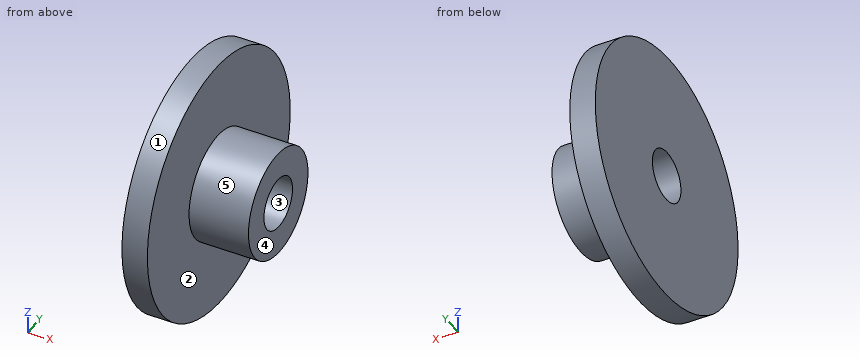
```python
from build123d import *

# Parameters (mm, degrees)
SKETCH1_R           = 30
BOSS_EXTRUDE1_DEPTH = 3
SKETCH2_R           = 12.5
BOSS_EXTRUDE2_DEPTH = 14
SKETCH3_R           = 6
CUT_EXTRUDE1_DEPTH  = 47.904157598


with BuildPart() as part:
    # Sketch1 → Boss-Extrude1 (new, symmetric)
    with BuildSketch(Plane(origin=(0, 0, 0), x_dir=(0, 0, -1), z_dir=(1, 0, 0))):
        Circle(SKETCH1_R)
    extrude(amount=BOSS_EXTRUDE1_DEPTH, both=True)

    # Sketch2 → Boss-Extrude2 (add)
    with BuildSketch(Plane(origin=(3, 0, 0), x_dir=(0, 0, -1), z_dir=(1, 0, 0))):
        Circle(SKETCH2_R)
    extrude(amount=BOSS_EXTRUDE2_DEPTH)

    # Sketch3 → Cut-Extrude1 (cut, through all)
    with BuildSketch(Plane(origin=(17, 0, 0), x_dir=(0, 0, -1), z_dir=(1, 0, 0))):
        Circle(SKETCH3_R)
    extrude(amount=-CUT_EXTRUDE1_DEPTH, mode=Mode.SUBTRACT)


solid = part.part
```
The listing builds one solid part. Answer for the finished solid, in the listing's coordinates (mm). Face numbers are marked on the shaded views. A direction names the side the tool comes from. Round coordinates to 2 decimals unless told otherwise and drop trailing zeros. Order: outer loops, then holes, each group sorted by start corner. A loop starts at its lowest first (then second) coordinate and runs counter-clockwise, first axis right, second up. Notation, with made-up numbers: (30, -31.75) - (54, -31.75) arc R26 ccw to (54, -0.75) - close; hole circle Ø4 at (60.25, 38). An arc over 180 degrees is marked (long way). Put each result on its own line as item: value. Start each with the question number.
(1) Find section D-D (z = -10.5). Give the vertices of the cut face in (x, y).
(2) Given P1, Ø3, axis at x = 1.5, z = -16, coming from the +Y side; P2, Ø8, axis at y = -13.5, z = -2.5, coming from the +X side; P3, Ø4, axis at x = 6.5, z = 2.5, coming from the -Y side; P4, Ø2, axis at x = 1, y = -11, coming from the +Z side, each flat-ended and moving along its own axis, determine where each tip first touches the part or whether it passes through.
(3) Find section A-A (z = 0). Give the vertices of the cut face in (x, y).
(4) For the marked faces 1 and 2, determine the directions among +Z, -Z, +X, -X, +Y, -Y from which every point of the face is accessible in a straight line to the end or side of a thin tool.
(5) Determine the mould class of the marked faces 3, 4 and 5 for opening direction Y: released by +Y, released by -Y, zero draft, split by the parting line, or undercut.
(6) Find section C-C (x = 14.75). Give the vertices of the cut face in (y, z), plus the area to 3 significant figures.
(7) Straight lines are drawn through the part: probe 1 along Y at (x, z) = (9.75, 0); probe 2 along X at (y, z) = (15.5, 16); probe 3 along Z at (x, y) = (4.5, -0.5). For each, find the intervals that lie inside material, in ascending order. Write a range as from..to.
Reply:
1. outline: (-3, -28.1) - (3, -28.1) - (3, -6.78) - (17, -6.78) - (17, 6.78) - (3, 6.78) - (3, 28.1) - (-3, 28.1) - close
2. P1: y = 26.26
2. P2: x = 17
2. P3: y = -12.49
2. P4: z = 28.28
3. outline: (-3, -30) - (3, -30) - (3, -12.5) - (17, -12.5) - (17, -6) - (-3, -6) - close; (-3, 6) - (17, 6) - (17, 12.5) - (3, 12.5) - (3, 30) - (-3, 30) - close
4. face 1: +X, -X
4. face 2: +X
5. face 3: undercut
5. face 4: zero draft
5. face 5: split by the parting line
6. outline: circle Ø25 at (0, 0); hole circle Ø12 at (0, 0)
6. area: 378 mm^2
7. probe 1: -12.5..-6, 6..12.5
7. probe 2: -3..3
7. probe 3: -12.49..-5.98, 5.98..12.49
